Autodesk Inventor part; units mm, degrees
ref_plane "YZ Plane" through (0, 0, 0) normal (1, 0, 0) x (0, 1, 0)
ref_plane "XZ Plane" through (0, 0, 0) normal (0, 1, 0) x (-1, 0, 0)
ref_plane "XY Plane" through (0, 0, 0) normal (0, 0, 1) x (1, 0, 0)
sketch "Sketch1" plane through (0, 0, 0) normal (0, 0, 1) x (1, 0, 0)
  line L0 (0, 0) -> (-224.5064, 224.5064)
  line L1 (0, 0) -> (317.5, 0) construction
  line L2 (-224.5064, 224.5064) -> (-262.6064, 224.5064)
  line L3 (-262.6064, 224.5064) -> (-262.6064, 211.8064)
  line L4 (-262.6064, 211.8064) -> (-229.7669, 211.8064)
  line L5 (-229.7669, 211.8064) -> (-224.5064, 224.5064)
  line L6 (0, 0) -> (-8.9803, -8.9803)
  line L7 (-8.9803, -8.9803) -> (-229.7669, 211.8064)
  line L8 (0, 0) -> (-1.1225, -1.1225)
  line L9 (-1.1225, -1.1225) -> (-225.164, 222.9189)
  line L10 (-262.6064, 224.5064) -> (-262.6064, 222.9189)
  line L11 (-262.6064, 222.9189) -> (-225.164, 222.9189)
  dimension "d0" = 317.5
  dimension "d1" = 135
  dimension "d2" = 38.1
  dimension "d3" = 12.7
  dimension "d5" = 12.7
  dimension "d6" = 90
  dimension "d9" = 1.5875
  dimension "d10" = 1.5875
  dimension "d11" = 90
extrude "Extrusion1" add sketch "Sketch1" along normal blind 1.5875
extrude "Extrusion3" add sketch "Sketch1" against normal blind 11.1125 contours L5 L11 L3 L2
extrude "Extrusion4" add sketch "Sketch1" against normal blind 11.1125 contours L6 L9 L5 L0
properties part number "DiagL"
Source: CAD feature listing. Evaluate the final solid. Frame: model axes, mm. A direction names the side the tool comes from. Round coordinates to 2 decimals unless told otherwise and drop trailing zeros. Loops run counter-clockwise (first coordinate to the right, second up) from the corner with the lowest first, then second, coordinate; pieces in that order, holes last. Notation, with made-up numbers: M 5.5,74 L 60.5,74 A34 cw 60.5,110 Z; hole C 53,2 d10. An arc over 180 degrees is marked long. Use a Markdown table: item, result. Add a question column.
1. Cut plane A-A, the plane z = -5. Output: boundary loops of the cut face in (x, y).
2. Ray query, line 1 along Z through (x, y) = (-66, 59); line 2 along Y through (x, z) = (-231, 1.25); line 3 along Y through (x, z) = (-228, -8). Return the intervals inside material, ascending. Write a range as [from, to].
3. Set-up query: faces 1 (the flat face through (-111, 111, -5)), 2 (the flat face through (-244, 222.919, -5)). Return all of +Z, -Z, +X, -X, +Y, -Y with unobstructed straight access to the full face (end or side cutting, diameter ignored); none if empty.
4. Contact query for flat-ended pins moving along their axis: pin 1 (3 mm diameter, centred on x = -162, z = -4, fed in from +Y); pin 2 (6 mm diameter, centred on y = 153, z = -9.5, fed in from +X); pin 3 (1.5 mm diameter, centred on y = 138.5, z = -5, fed in from -X). Output: stop coordinate, or through.
5. Cut plane B-B, the plane y = 121. Output: boundary loops of the cut face in (x, z).
Solution:
| question | item | result |
|---|---|---|
| 1 | outline | M -262.61,222.92 L -225.16,222.92 L -1.12,-1.12 L 0,0 L -224.51,224.51 L -262.61,224.51 Z |
| 2 | line 1 | z = [0, 1.59] |
| 2 | line 2 | y = [211.81, 224.51] |
| 2 | line 3 | y = [222.92, 224.51] |
| 3 | face 1 | +Z, -Z, +X, +Y |
| 3 | face 2 | -Z, -X, -Y |
| 4 | pin 1 | stops at y = 163.5 |
| 4 | pin 2 | stops at x = -150 |
| 4 | pin 3 | stops at x = -141.5 |
| 5 | outline | M -138.96,0 L -123.25,0 L -123.25,-11.11 L -121,-11.11 L -121,1.59 L -138.96,1.59 Z |
